Verification items for the finished model (mm, model axes). Coordinates: 2 decimals unless noted, no trailing zeros. Write each loop counter-clockwise with the first axis right and the second up, starting at its lowest first coordinate (ties: lowest second). Pieces come first, ordered by that corner, then holes. Notation, with made-up numbers: (60.25, 69.25) -> (96.25, 69.25) arc R24 ccw to (96.25, 93.25) -> close; hole circle Ø5 at (-7.5, -31.75). An arc over 180 degrees is marked (long way). Write item = value, one per line. Start each with the question number.
(1) Material ranges on probe 1 along Y at (x, z) = (0.55, -152); probe 2 along Y at (x, z) = (-0.85, -21.5); probe 3 along Y at (x, z) = (-0.55, -278), recorded low to high. Write a range as [from, to].
(2) Section check B-B (z = -135). Record the cut outline in (x, y).
(3) Gauge pin test, flat ends, axial feed: pin 1 Ø1.5 at (x, z) = (0.5, -422) entering from -Y; pin 2 Ø1.3 at (x, y) = (0.5, -8.5) entering from -Z. Record the tip position at first contact, or that the pin passes through.
(4) Section check D-D (y = -48.5). Record the cut outline in (x, z).
(5) Section check C-C (x = -0.4). State how many separate pieces and enclosed holes the cut face has, plus the area to 3 significant figures.
(6) Section check A-A (z = -402.5). Record the cut outline in (x, y), plus the area to 3 significant figures.
(7) Mould release check, pull along Z, two halves, no side actions. Record for faces 1 (the face through (1.5, -11, -180)), 2 (the face through (0.021, 23.642, -236.677)), 3 (the face through (-0.021, -71.517, -104.062)): released by +Z, released by -Z, zero draft, split by the parting line, or undercut.
```python
from build123d import *

# Parameters (mm, degrees)
BOSS_EXTRUDE1_DEPTH      = 1.5
BOSS_EXTRUDE1_DEPTH_BACK = 1.5
SKETCH3_W                = 152
SKETCH3_H                = 8.6
CUT_EXTRUDE1_DEPTH       = 520.533194562
FILLET1_R                = 3
SKETCH4_R                = 19.119387796
SKETCH4_R_2              = 47.191393473
SKETCH4_R_3              = 35.18699184
SKETCH4_R_4              = 12.586978738
SKETCH4_R_5              = 11.189603354
SKETCH4_R_6              = 21.557380713
CUT_EXTRUDE2_DEPTH       = 10


with BuildPart() as part:
    # Sketch2 → Boss-Extrude1 (new, two sides: drawn at the far end of the back side and taken through both)
    with BuildSketch(Plane(origin=(0, 0, 0), x_dir=(0, 0, -1), z_dir=(1, 0, 0)).offset(-BOSS_EXTRUDE1_DEPTH_BACK)):
        Polygon((0, 67.22485033), (205.165503831, 48.288859026), (513.4, -0.530689138), (513.4, -22.650154351), (205.250409944, -63.717607751), (0, -79.537288439), (-70, -79.537288439), (-70, -69.537288439), (0, 17.22485033), align=None)
    extrude(amount=BOSS_EXTRUDE1_DEPTH + BOSS_EXTRUDE1_DEPTH_BACK)

    # Sketch3 → Cut-Extrude1 (cut, through all)
    with BuildSketch(Plane(origin=(1.5, 0, 0), x_dir=(0, 0, -1), z_dir=(1, 0, 0))):
        with Locations((443.4, -8.3)):
            Rectangle(SKETCH3_W, SKETCH3_H)
    extrude(amount=-CUT_EXTRUDE1_DEPTH, mode=Mode.SUBTRACT)

    # Fillet1
    fillet1_edges = [part.edges().sort_by_distance(p)[0] for p in [
        (0, -12.6, -367.4),
        (0, -4, -367.4),
    ]]
    fillet(fillet1_edges, radius=FILLET1_R)

    # Sketch4 → Cut-Extrude2 (cut)
    with BuildSketch(Plane(origin=(1.5, 0, 0), x_dir=(0, 0, -1), z_dir=(1, 0, 0))):
        with Locations((-22.865600385, -55.069339131)):
            Circle(SKETCH4_R)
        with Locations((55.752747866, -6.379566635)):
            Circle(SKETCH4_R_2)
        with Locations((268.826339435, -6.379566635)):
            Circle(SKETCH4_R_3)
        with Locations((225.050213704, 28.462655886)):
            Circle(SKETCH4_R_4)
        with Locations((17.336964062, 48.563938109)):
            Circle(SKETCH4_R_5)
        with Locations((225.050213704, -40.775093995)):
            Circle(SKETCH4_R_4)
        with Locations((327.790100624, -26.927544019)):
            Circle(SKETCH4_R_4)
        with Locations((327.790100624, 9.701459144)):
            Circle(SKETCH4_R_4)
        with Locations((149.867646424, 23.293890716)):
            Circle(SKETCH4_R_6)
        with Locations((149.867646424, -35.180680846)):
            Circle(SKETCH4_R_6)
    extrude(amount=-CUT_EXTRUDE2_DEPTH, mode=Mode.SUBTRACT)


solid = part.part
```
Response:
q1.probe_1 = [-67.82, -56.63], [-13.73, 1.84], [44.75, 53.2]
q1.probe_2 = [-77.88, -38.84], [26.08, 38.18], [58.95, 65.24]
q1.probe_3 = [-54.02, -40.35], [27.59, 36.75]
q2.outline = (-1.5, -69.13) -> (1.5, -69.13) -> (1.5, -50.79) -> (-1.5, -50.79) -> close; (-1.5, -19.57) -> (1.5, -19.57) -> (1.5, 7.68) -> (-1.5, 7.68) -> close; (-1.5, 38.9) -> (1.5, 38.9) -> (1.5, 54.76) -> (-1.5, 54.76) -> close
q3.pin_1 = -34.93
q3.pin_2 = -367.4
q4.outline = (-1.5, -319.44) -> (1.5, -319.44) -> (1.5, -234.99) -> (-1.5, -234.99) -> close; (-1.5, -215.11) -> (1.5, -215.11) -> (1.5, -166.82) -> (-1.5, -166.82) -> close; (-1.5, -132.92) -> (1.5, -132.92) -> (1.5, -77.03) -> (-1.5, -77.03) -> close; (-1.5, -34.47) -> (1.5, -34.47) -> (1.5, 4.91) -> (-1.5, 4.91) -> close; (-1.5, 40.82) -> (1.5, 40.82) -> (1.5, 53.03) -> (-1.5, 53.03) -> close
q5.separate_pieces = 1
q5.enclosed_holes = 10
q5.area = 32,400 mm2
q6.outline = (-1.5, -37.43) -> (1.5, -37.43) -> (1.5, -12.6) -> (-1.5, -12.6) -> close; (-1.5, -4) -> (1.5, -4) -> (1.5, 17.03) -> (-1.5, 17.03) -> close
q6.area = 138 mm2
q7.face_1 = zero draft
q7.face_2 = undercut
q7.face_3 = released by -Z
